Design review of the part shown in the three views and the two pictorial views. Dimensions are in mm from the part's minimum x, y and z. A direction names the side the tool comes from. Give positions to 0.01 mm unless a question says otherwise; leave off trailing zeros. Order: outer loops, then holes, each group sorted by start corner. A loop starts at its lowest first (then second) coordinate and runs counter-clockwise, first axis right, second up.
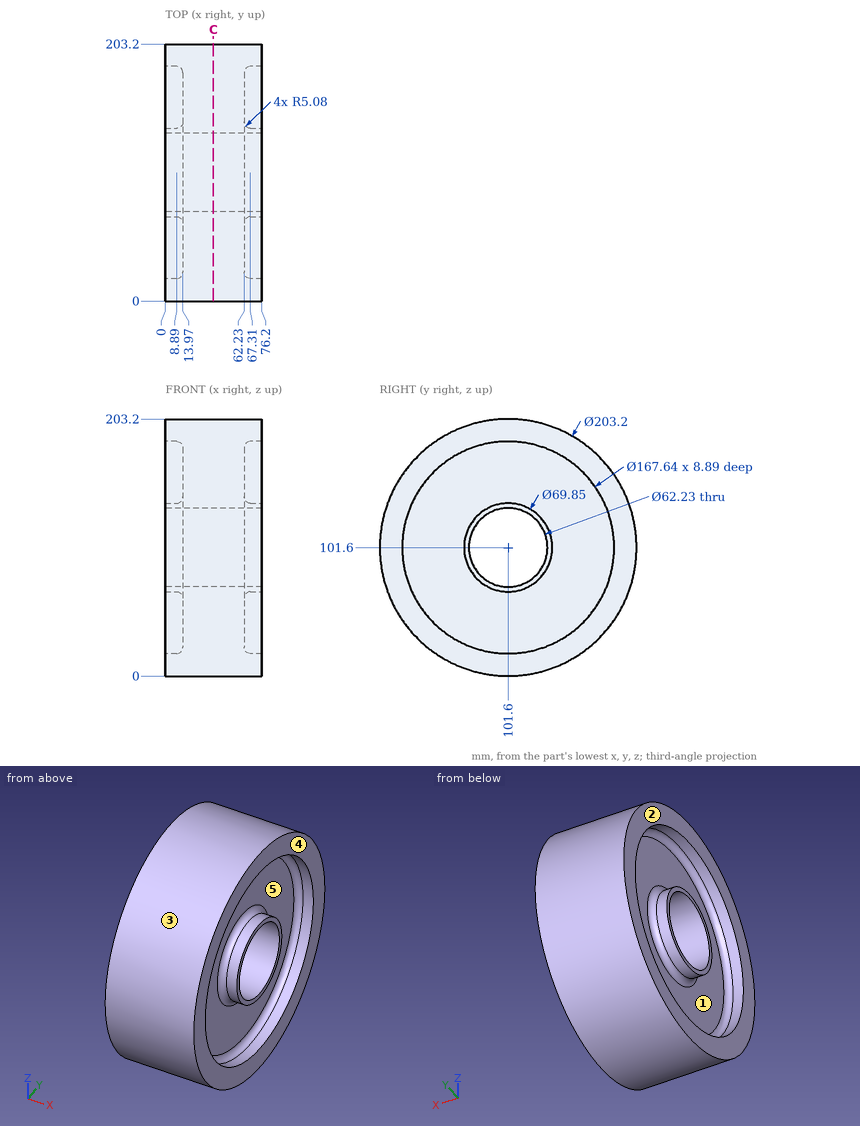
Item 1: Take a section at C-C (x = 38). Give the boundary of the cut face in (y, z) (3 decimals).
Values found:
outline: circle Ø203.2 at (101.6, 101.6); hole circle Ø62.23 at (101.6, 101.6)
Item 2: Draft analysis for pull direction Y (two halves, no side actions). For the marked faces 1, 2 and 3, state which applies: released by +Y, released by -Y, zero draft, split by the parting line, or undercut.
Values found:
face 1: undercut
face 2: zero draft
face 3: split by the parting line
Item 3: Clearance check with flat-ended pins moving along their axes: pin 1 Ø12 at (x, z) = (38.5, 29.5) entering from -Y; pin 2 Ø2 at (x, z) = (56, 46) entering from -Y; pin 3 Ø5 at (y, z) = (157.5, 94) entering from +X. State where each tip first meets the part, or that it passes through.
Values found:
pin 1: stops at y = 24.44
pin 2: stops at y = 15.92
pin 3: stops at x = 62.23
Item 4: For the marked faces 4 and 5, list the 3-axis set-ups (+Z, -Z, +X, -X, +Y, -Y) from which the entire face can be reached by the end or side of a thin tool; tool diameter is ignored.
Values found:
face 4: +Z, -Z, +X, +Y, -Y
face 5: +X
Item 5: For line 1 (Z direction, x = 74.25, y = 101.6) (3 decimals); line 2 (Z direction, x = 20, y = 101.6) (3 decimals); line 3 (X direction, y = 97.5, z = 159.5), list the stretches that pass through material, from the lowest coordinate up.
Values found:
line 1: z = 0 to 17.78, 66.675 to 70.485, 132.715 to 136.525, 185.42 to 203.2
line 2: z = 0 to 70.485, 132.715 to 203.2
line 3: x = 13.97 to 62.23
